```python
from build123d import *

# Parameters (mm, degrees)
SKETCH1_W          = 12.617819502
SKETCH1_H          = 2
SKETCH1_W_2        = 6.5532
SKETCH1_H_2        = 7.545
SKETCH2_R          = 26.652766262
SKETCH2_R_2        = 14.565
CUT_EXTRUDE1_DEPTH = 10
SKETCH4_R          = 1.0922
CUT_EXTRUDE2_DEPTH = 30.490976315


with BuildPart() as part:
    # Sketch1 → Revolve1 (revolve)
    with BuildSketch(Plane(origin=(0, 0, 0), x_dir=(1, 0, 0), z_dir=(0, 1, 0))):
        with Locations((-13.308909751, 3.700473465)):
            Rectangle(SKETCH1_W, SKETCH1_H)
        Polygon((-11.938, 2.700473465), (-19.617819502, 2.700473465), (-19.617819502, -0.474526535), (-13.064619502, -0.474526535), (-11.938, -0.474526535), align=None)
        with Locations((-16.341219502, -4.247026535)):
            Rectangle(SKETCH1_W_2, SKETCH1_H_2)
    revolve(axis=Axis((0, 0, -25.411285606), (0, 0, 1)))

    # Sketch2 → Cut-Extrude1 (cut)
    with BuildSketch(Plane(origin=(0, 0, -4.700473465), x_dir=(-1, 0, 0), z_dir=(0, 0, -1))):
        Circle(SKETCH2_R)
        Circle(SKETCH2_R_2, mode=Mode.SUBTRACT)
    extrude(amount=-CUT_EXTRUDE1_DEPTH, mode=Mode.SUBTRACT)

    # Sketch4 → Cut-Extrude2 (cut, through all)
    with BuildSketch(Plane(origin=(0, 0, 5.299526535), x_dir=(-1, 0, 0), z_dir=(0, 0, -1))):
        with Locations((16.57, 0)):
            Circle(SKETCH4_R)
        with Locations(Location((-16.57, 0, 0), (0, 0, 180))):
            Circle(SKETCH4_R)
    extrude(amount=-CUT_EXTRUDE2_DEPTH, mode=Mode.SUBTRACT)


solid = part.part
```
Design review of the part built by this model. Coordinates are the model's own, in mm. A direction names the side the tool comes from. Coordinates: 2 decimals unless noted, no trailing zeros. Loops run counter-clockwise (first coordinate to the right, second up) from the corner with the lowest first, then second, coordinate; pieces in that order, holes last. Notation, with made-up numbers: M 32.25,-24.75 L 61.25,-24.75 A16 cw 61.25,2.25 Z; hole C -21,5.5 d8. An arc over 180 degrees is marked long. One line per question, with ' | ' between items.
(1) We need section C-C (y = 5.5). Give the boundary of the cut face in (x, z), and give its area (3 significant figures).
Filled in:
outline: M -18.83,5.3 L -13.49,5.3 L -13.49,-4.7 L -4.33,-4.7 L -4.33,-2.7 L -10.6,-2.7 L -10.6,0.47 L -11.85,0.47 L -11.85,8.02 L -18.83,8.02 Z; M 4.33,-4.7 L 13.49,-4.7 L 13.49,5.3 L 18.83,5.3 L 18.83,8.02 L 11.85,8.02 L 11.85,0.47 L 10.6,0.47 L 10.6,-2.7 L 4.33,-2.7 Z | area: 109 mm^2
(2) Wall thickness on probe 1 along Y at (x, z) = (0, 6); probe 2 along Y at (x, z) = (0, -0.85) (3 decimals); probe 3 along Z at (x, y) = (5, -11): over which ranges is each line inside the solid? List them lowest first.
Filled in:
probe 1: y = -19.62 to -13.06, 13.06 to 19.62 | probe 2: y = -14.565 to -11.938, 11.938 to 14.565 | probe 3: z = -4.7 to 0.47
(3) For pin 1 Ø4 at (x, z) = (-7, 6.5) entering from +Y; pin 2 Ø1.3 at (x, y) = (16.57, 0) entering from +Z; pin 3 Ø1.5 at (y, z) = (6.5, 4.5) entering from +X; pin 4 Ø3 at (y, z) = (-8, -1) entering from +X, all flat-tipped, find the tip position at first contact; note any pin that passes through.
Filled in:
pin 1: stops at y = 18.97 | pin 2: passes through | pin 3: stops at x = 13.38 | pin 4: stops at x = 13.03
(4) We need section A-A (x = 0). Give the boundary of the cut face in (y, z) (3 decimals).
Filled in:
outline: M -19.618,5.3 L -14.565,5.3 L -14.565,-4.7 L -7,-4.7 L -7,-2.7 L -11.938,-2.7 L -11.938,0.475 L -13.065,0.475 L -13.065,8.02 L -19.618,8.02 Z; M 7,-4.7 L 14.565,-4.7 L 14.565,5.3 L 19.618,5.3 L 19.618,8.02 L 13.065,8.02 L 13.065,0.475 L 11.938,0.475 L 11.938,-2.7 L 7,-2.7 Z
(5) We need section B-B (y = 0). Give the boundary of the cut face in (x, z) (3 decimals), and give its area (3 significant figures).
Filled in:
outline: M -19.618,5.3 L -17.662,5.3 L -17.662,8.02 L -19.618,8.02 Z; M -15.478,5.3 L -14.565,5.3 L -14.565,-4.7 L -7,-4.7 L -7,-2.7 L -11.938,-2.7 L -11.938,0.475 L -13.065,0.475 L -13.065,8.02 L -15.478,8.02 Z; M 7,-4.7 L 14.565,-4.7 L 14.565,5.3 L 15.478,5.3 L 15.478,8.02 L 13.065,8.02 L 13.065,0.475 L 11.938,0.475 L 11.938,-2.7 L 7,-2.7 Z; M 17.662,5.3 L 19.618,5.3 L 19.618,8.02 L 17.662,8.02 Z | area: 85.2 mm^2
(6) Draft analysis for pull direction Y (two halves, no side actions). For faces 1 (the face through (-4, 13, 8.02)), 2 (the face through (2.55, -19.45, 6.68)), 3 (the face through (-5.1, 5.1, -2.7)), state which applies: released by +Y, released by -Y, zero draft, split by the parting line, or undercut.
Filled in:
face 1: zero draft | face 2: split by the parting line | face 3: undercut
(7) We need section D-D (z = 6.5). Give the boundary of the cut face in (x, y), and give its area (3 significant figures).
Filled in:
outline: C 0,0 d39.24; hole C -16.57,0 d2.18; hole C 0,0 d26.13; hole C 16.57,0 d2.18 | area: 665 mm^2
(8) Machinability: for faces 4 (the face through (-6.466, 2.681, -3.714)), 5 (the face through (0, 15, 5.3)), 6 (the face through (2.588, 11.654, -1.135)), which of the approach directions +Z, -Z, +X, -X, +Y, -Y give a long, thin tool a straight path to every point of the face, cutting with its end or side? Answer none if there is none.
Filled in:
face 4: +Z, -Z | face 5: -Z | face 6: +Z
